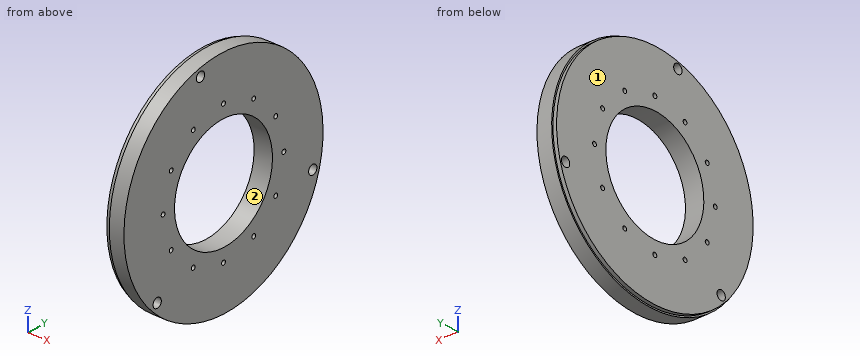
```python
from build123d import *

# Parameters (mm, degrees)
SKETCH1_R           = 76.2
BOSS_EXTRUDE1_DEPTH = 12.7
SKETCH2_R           = 37.5
CUT_EXTRUDE1_DEPTH  = 109.508847566
SKETCH8_R           = 1.4732
CUT_EXTRUDE3_DEPTH  = 109.508847566
CIRPATTERN6_COUNT   = 12
SKETCH11_R          = 3.175
CUT_EXTRUDE4_DEPTH  = 109.508847566
CIRPATTERN7_COUNT   = 3
SKETCH13_OUTSIDE_W  = 197.58
SKETCH13_OUTSIDE_H  = 197.58
SKETCH13_OUTSIDE_R  = 75.2221
CUT_EXTRUDE5_DEPTH  = 2.54


with BuildPart() as part:
    # Sketch1 → Boss-Extrude1 (new body)
    with BuildSketch(Plane(origin=(0, 0, 0), x_dir=(0, 0, -1), z_dir=(1, 0, 0))):
        Circle(SKETCH1_R)
    extrude(amount=BOSS_EXTRUDE1_DEPTH)

    # Sketch2 → Cut-Extrude1 (cut, through all)
    with BuildSketch(Plane(origin=(12.7, 0, 0), x_dir=(0, 0, -1), z_dir=(1, 0, 0))):
        Circle(SKETCH2_R)
    extrude(amount=-CUT_EXTRUDE1_DEPTH, mode=Mode.SUBTRACT)

    # Sketch8 → Cut-Extrude3 (cut, through all)
    with BuildSketch(Plane(origin=(12.7, 0, 0), x_dir=(0, 0, -1), z_dir=(1, 0, 0))):
        with Locations((0, 46.228)):
            Circle(SKETCH8_R)
    cut_extrude3 = extrude(amount=-CUT_EXTRUDE3_DEPTH, mode=Mode.SUBTRACT)

    # CirPattern6: Cut-Extrude3 ×12 about axis
    cirpattern6_axis = Axis((0, 0, 0), (1, 0, 0))
    for i in range(1, CIRPATTERN6_COUNT):
        add(cut_extrude3.rotate(cirpattern6_axis, i * 360 / CIRPATTERN6_COUNT), mode=Mode.SUBTRACT)

    # Sketch11 → Cut-Extrude4 (cut, through all)
    with BuildSketch(Plane(origin=(12.7, 0, 0), x_dir=(0, 0, -1), z_dir=(1, 0, 0))):
        with Locations((19.159653756, 68.353359348)):
            Circle(SKETCH11_R)
    cut_extrude4 = extrude(amount=-CUT_EXTRUDE4_DEPTH, mode=Mode.SUBTRACT)

    # CirPattern7: Cut-Extrude4 ×3 about axis
    cirpattern7_axis = Axis((0, 0, 0), (1, 0, 0))
    for i in range(1, CIRPATTERN7_COUNT):
        add(cut_extrude4.rotate(cirpattern7_axis, i * 360 / CIRPATTERN7_COUNT), mode=Mode.SUBTRACT)

    # Sketch13 outside → Cut-Extrude5 (cut)
    with BuildSketch(Plane.ZY):
        Rectangle(SKETCH13_OUTSIDE_W, SKETCH13_OUTSIDE_H)
        Circle(SKETCH13_OUTSIDE_R, mode=Mode.SUBTRACT)
    extrude(amount=-CUT_EXTRUDE5_DEPTH, mode=Mode.SUBTRACT)


solid = part.part
```
Design review of the part built by this model. Coordinates are the model's own, in mm. Face numbers are marked on the shaded views. Coordinates: 2 decimals unless noted, no trailing zeros. Order: outer loops, then holes, each group sorted by start corner. A loop starts at its lowest first (then second) coordinate and runs counter-clockwise, first axis right, second up.
1) Wall thickness on line 1 along Y through (x, z) = (4.5, 0); line 2 along Z through (x, y) = (6.75, 39); line 3 along Y through (x, z) = (4, 23): over which ranges is each line inside the solid? List them lowest first.
2) Clearance check with flat-ended pins moving along their axes: pin 1 (1 mm diameter, centred on x = 10, y = 51.5, fed in from -Z); pin 2 (6 mm diameter, centred on x = 10, y = -43, fed in from -Z); pin 3 (3 mm diameter, centred on x = 3.5, z = 1, fed in from +Y). State where each tip first meets the part, or that it passes through.
3) Take a section at D-D, the plane z = -56.5. Give the boundary of the cut face in (x, y), and give its area (3 significant figures).
4) Take a section at B-B, the plane y = -66.5. Give the boundary of the cut face in (x, z).
5) Mouldability with a two-part tool opening along Y and no side actions: class the marked faces 1 and 2 as +Y half, -Y half, draft (parallel to the pull), parting line (faces both ways), or undercut.
6) Take a section at C-C, the plane x = 5. State how many separate pieces and enclosed holes the cut face has, and give its area (3 significant figures).
7) Take a section at A-A, the plane z = 12. Give the boundary of the cut face in (x, y), and give its area (3 significant figures).
Returned:
1. line 1: y = -76.2 to -47.7, -44.75 to -37.5, 37.5 to 44.75, 47.7 to 76.2
1. line 2: z = -65.46 to -24.16, -22.07 to 22.07, 24.16 to 65.46
1. line 3: y = -72.65 to -41.5, -38.57 to -29.62, 29.62 to 38.57, 41.5 to 72.65
2. pin 1: stops at z = -56.62
2. pin 2: stops at z = -64.86
2. pin 3: stops at y = 76.2
3. outline: (0, -49.66) - (2.54, -49.66) - (2.54, -51.13) - (12.7, -51.13) - (12.7, 51.13) - (2.54, 51.13) - (2.54, 49.66) - (0, 49.66) - close
3. area: 1,290 mm2
4. outline: (0, -35.16) - (2.54, -35.16) - (2.54, -37.2) - (12.7, -37.2) - (12.7, 37.2) - (2.54, 37.2) - (2.54, 35.16) - (0, 35.16) - close
5. face 1: draft
5. face 2: undercut
6. separate pieces: 1
6. enclosed holes: 16
6. area: 13,600 mm2
7. outline: (0, -74.26) - (2.54, -74.26) - (2.54, -75.25) - (12.7, -75.25) - (12.7, -35.53) - (0, -35.53) - close; (0, 35.53) - (12.7, 35.53) - (12.7, 75.25) - (2.54, 75.25) - (2.54, 74.26) - (0, 74.26) - close
7. area: 1,000 mm2
